Source: three-view drawing plus pictorial views. Frame: mm from the lowest corner of the part. A direction names the side the tool comes from. Give positions to 0.01 mm unless a question says otherwise; leave off trailing zeros. Loops run counter-clockwise (first coordinate to the right, second up) from the corner with the lowest first, then second, coordinate; pieces in that order, holes last. Notation, with made-up numbers: M 13,-13 L 53,-13 A16 cw 53,14 Z; hole C 5.25,23 d3. An arc over 180 degrees is marked long. One line per item, written item: value. Start each with the question number.
(1) Pull-direction query (Z, two-part tool) for the marked faces 3 and 4; classes: released by +Z, released by -Z, zero draft, split by the parting line, or undercut.
(2) Section A-A on z = 50.9. Output: boundary loops of the cut face in (x, y), plus the area to 3 significant figures.
(3) Section B-B on y = 17.75. Output: boundary loops of the cut face in (x, z), plus the area to 3 significant figures.
(4) Access query for the marked faces 1 and 2. Directions: +Z, -Z, +X, -X, +Y, -Y. A direction counts if a zero-diameter tool reaches every point of the face in a straight line with its end or side. Return the directions, or none.
(5) Section C-C on y = 11.25. Output: boundary loops of the cut face in (x, z).
(6) Pin query (flat end, axial travel): P1, Ø4, axis at x = 20.5, y = 5.5, coming from the -Z side; P2, Ø4, axis at x = 32, y = 9.5, coming from the -Z side; P3, Ø12, axis at x = 34.5, z = 47.5, coming from the +Y side. Return the tip coordinate at first contact, or that it passes through.
(7) Ray query, line 1 along Z through (x, y) = (50.9, 7); line 2 along Z through (x, y) = (50.9, 13.3); line 3 along Y through (x, z) = (20.5, 55.5). Return the intervals inside material, ascending. Write a range as from..to.
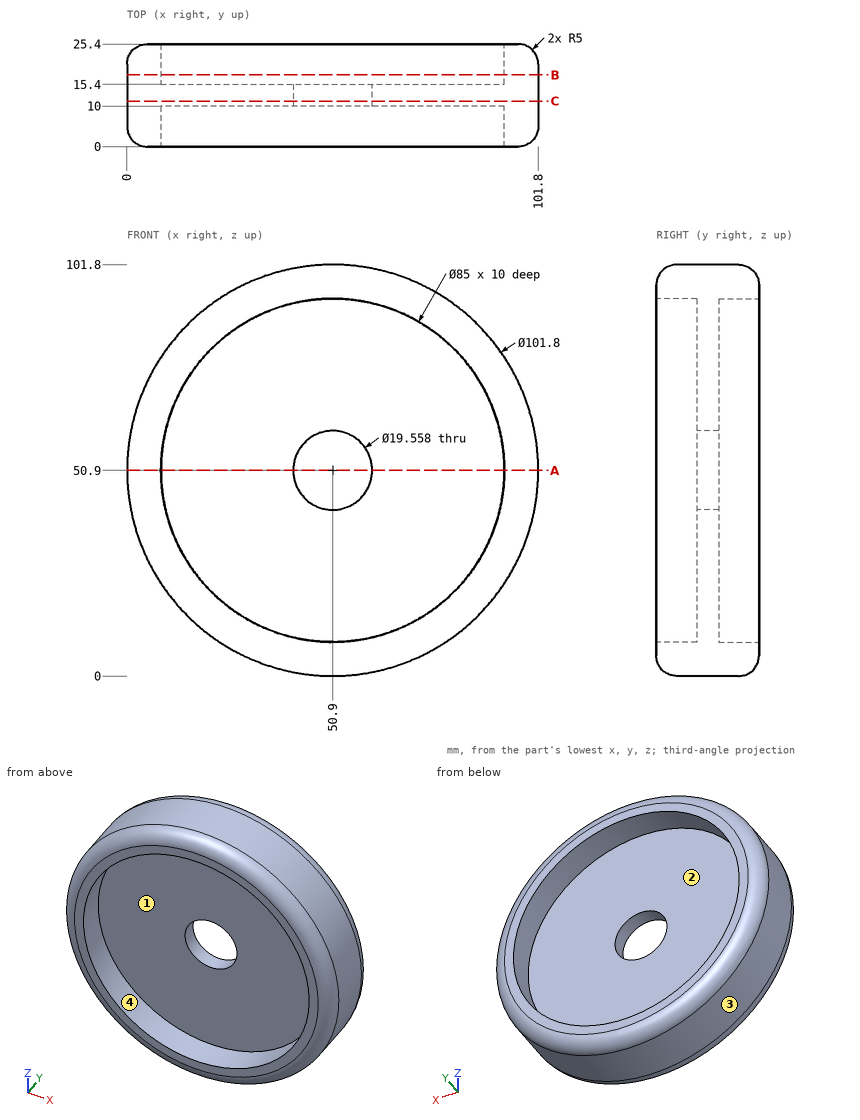
Output values:
1. face 3: split by the parting line
1. face 4: undercut
2. outline: M 0,5 A5 ccw 5,0 L 8.4,0 L 8.4,10 L 41.12,10 L 41.12,15.4 L 8.4,15.4 L 8.4,25.4 L 5,25.4 A5 ccw 0,20.4 Z; M 60.68,10 L 93.4,10 L 93.4,0 L 96.8,0 A5 ccw 101.8,5 L 101.8,20.4 A5 ccw 96.8,25.4 L 93.4,25.4 L 93.4,15.4 L 60.68,15.4 Z
2. area: 759 mm²
3. outline: C 50.9,50.9 d101.8; hole C 50.9,50.9 d85
3. area: 2,460 mm²
4. face 1: -Y
4. face 2: +Y
5. outline: C 50.9,50.9 d101.8; hole C 50.9,50.9 d19.56
6. P1: stops at z = 8.66
6. P2: stops at z = 2.89
6. P3: stops at y = 15.4
7. line 1: z = 0..8.4, 93.4..101.8
7. line 2: z = 0..41.12, 60.68..101.8
7. line 3: y = 10..15.4
